Part model, mm, in its own coordinate system. A direction names the side the tool comes from. Give positions to 0.01 mm unless a question says otherwise; leave off trailing zeros. Loops run counter-clockwise (first coordinate to the right, second up) from the corner with the lowest first, then second, coordinate; pieces in that order, holes last. Notation, with made-up numbers: M 33.25,7 L 47.25,7 A12 cw 47.25,17 Z; hole C 17.5,20 d7. An arc over 180 degrees is marked long. Put each result on its own line as item: value. Start each with the question number.
```python
from build123d import *

# Parameters (mm, degrees)
F1_W     = 65.024
F1_H     = 21.336
F2_DEPTH = 4.7625
F1_H_2   = 4.7625
F3_DEPTH = 13.0175


# Not quite as in the source:
# - a variable given as a bare number and used for a length is read in inches; the dataset says mm whatever the document's units were


with BuildPart() as f2:
    # F1 (on Top) → F2 (new body)
    with BuildSketch(Plane.XY):
        Rectangle(F1_W, F1_H)
    extrude(amount=F2_DEPTH)

    # F1 (on Top) → F3 (join)
    with BuildSketch(Plane.XY):
        Polygon((37.2745, 15.4305), (-37.2745, 15.4305), (-37.2745, 10.668), (-32.512, 10.668), (32.512, 10.668), (37.2745, 10.668), align=None)
        Polygon((37.2745, -15.4305), (37.2745, 10.668), (32.512, 10.668), (32.512, -10.668), (32.512, -15.4305), align=None)
        with Locations((0, -13.04925)):
            Rectangle(F1_W, F1_H_2)
        Polygon((-32.512, 10.668), (-37.2745, 10.668), (-37.2745, -15.4305), (-32.512, -15.4305), (-32.512, -10.668), align=None)
    extrude(amount=F3_DEPTH)


solid = f2.part
```
1) Which spindle directions (+Z, -Z, +X, -X, +Y, -Y) get a long thin tool onto all of the face, cutting with end or side? Do faces 1 (the flat face through (32.512, 0, 9)), 2 (the flat face through (-1, 0, 0)). Say none if no direction does.
2) Band-saw the part on C-C on x = -30. Give the cut face in (y, z).
3) Band-saw the part on B-B on z = 6.75. Give the cut face in (x, y), then the cut area to 3 significant figures.
4) Wall check: L1, parallel to Y at x = -12, z = 9.5; L2, parallel to X at y = -1.5, z = 8.25; L3, parallel to Z at x = -25.5, y = -10.5. Give the ranges that are in metal, low to high.
5) Pin check, flat tip, straight feed: pin 1 Ø12 at (x, y) = (-11, 3.5) entering from +Z. Stop position of the tip, or through.
6) Mould opens along X. For faces 3 (the flat face through (37.274, 0, 6)), 4 (the flat face through (1, 15.43, 6)), 5 (the flat face through (0, 10.668, 9)) say: +X half, -X half, draft (parallel to the pull), parting line (faces both ways), or undercut.
7) Band-saw the part on A-A on y = -1.5. Give the cut face in (x, z).
Evaluation:
1. face 1: +Z
1. face 2: -Z, +X, -X, +Y, -Y
2. outline: M -15.43,0 L 15.43,0 L 15.43,13.02 L 10.67,13.02 L 10.67,4.76 L -10.67,4.76 L -10.67,13.02 L -15.43,13.02 Z
3. outline: M -37.27,-15.43 L 37.27,-15.43 L 37.27,15.43 L -37.27,15.43 Z; hole M -32.51,-10.67 L 32.51,-10.67 L 32.51,10.67 L -32.51,10.67 Z
3. area: 913 mm2
4. L1: -15.43 to -10.67, 10.67 to 15.43
4. L2: -37.27 to -32.51, 32.51 to 37.27
4. L3: 0 to 4.76
5. pin 1: z = 4.76
6. face 3: +X half
6. face 4: draft
6. face 5: undercut
7. outline: M -37.27,0 L 37.27,0 L 37.27,13.02 L 32.51,13.02 L 32.51,4.76 L -32.51,4.76 L -32.51,13.02 L -37.27,13.02 Z
